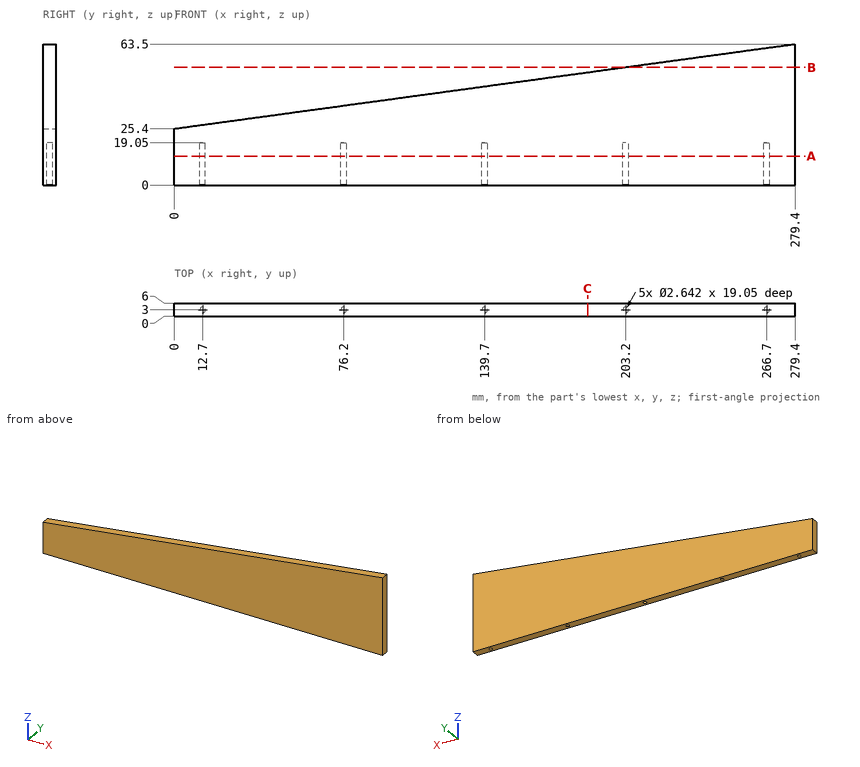
Can you work these out from the drawing? Everything is in mm from the part's minimum corner. Give positions to 0.01 mm unless a question says otherwise; leave off trailing zeros. Order: outer loops, then holes, each group sorted by start corner. A loop starts at its lowest first (then second) coordinate and runs counter-clockwise, first axis right, second up. Notation, with made-up numbers: M -19.5,-28.5 L 26.5,-28.5 A24 cw 26.5,-1.5 Z; hole C 71,-13 d7. An arc over 180 degrees is marked long. Use a Markdown table: item, result. Add a question column.
1. Suppose I cut it at A-A (z = 13). List the corners of the cut face in (x, y) for me, and give its area (3 significant figures).
2. Suppose I cut it at B-B (z = 53). List the corners of the cut face in (x, y) for me, and give its area (3 significant figures).
3. Suppose I cut it at C-C (x = 186). List the corners of the cut face in (y, z) for me.
4. I need wall thicknesses on probe 1 along Y at (x, z) = (203.2, 8.25); probe 2 along X at (y, z) = (3.55, 9.5); probe 3 along X at (y, z) = (1.95, 9) (1 decimal). Which ranges of each line are inside material? Lowest first, please. Write a range as from..to.
5. For pin 1 Ø1.3 at (x, y) = (12.5, 3) entering from -Z, with a flat end and sliding along its axis, tell me the tip position at first contact or that it passes through.
Results list:
| question | item | result |
|---|---|---|
| 1 | outline | M 0,0 L 279.4,0 L 279.4,6 L 0,6 Z; hole C 12.7,3 d2.64; hole C 76.2,3 d2.64; hole C 139.7,3 d2.64; hole C 203.2,3 d2.64; hole C 266.7,3 d2.64 |
| 1 | area | 1,650 mm² |
| 2 | outline | M 202.4,0 L 279.4,0 L 279.4,6 L 202.4,6 Z |
| 2 | area | 462 mm² |
| 3 | outline | M 0,0 L 6,0 L 6,50.76 L 0,50.76 Z |
| 4 | probe 1 | y = 0..1.68, 4.32..6 |
| 4 | probe 2 | x = 0..11.5, 13.9..75, 77.4..138.5, 140.9..202, 204.4..265.5, 267.9..279.4 |
| 4 | probe 3 | x = 0..11.9, 13.5..75.4, 77..138.9, 140.5..202.4, 204..265.9, 267.5..279.4 |
| 5 | pin 1 | stops at z = 19.05 |
